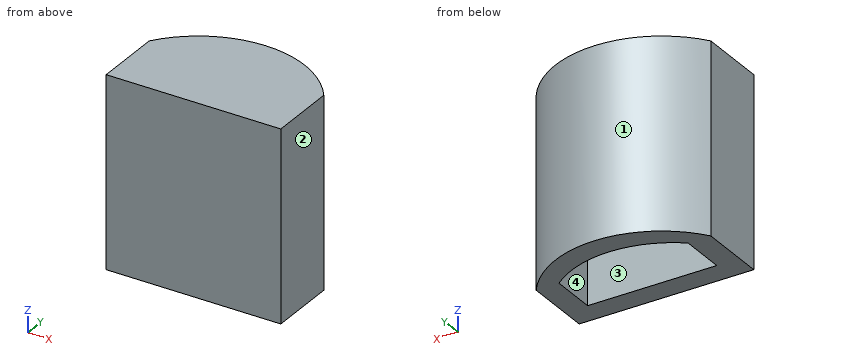
from build123d import *

# Parameters (mm, degrees)
EXTRUDE_1_DEPTH      = 5
EXTRUDE_2_DEPTH      = 5
EXTRUDE_2_DEPTH_BACK = 20


with BuildPart() as part:
    # 草圖1 → 填料-伸長1 (new body)
    with BuildSketch(Plane.XY):
        with BuildLine():
            Line((-8.181868209, 3.138333333), (-8.181868209, -2.861666667))
            Line((-8.181868209, -2.861666667), (8.818131791, -2.861666667))
            Line((8.818131791, -2.861666667), (8.818131791, 3.138333333))
            ThreePointArc((8.818131791, 3.138333333), (0.318131791, 6.138333333), (-8.181868209, 3.138333333))
        make_face()
    extrude(amount=EXTRUDE_1_DEPTH)

    # 草圖1<4> → 填料-伸長2 (add, two sides: drawn at the far end of the back side and taken through both)
    with BuildSketch(Plane.XY.offset(-EXTRUDE_2_DEPTH_BACK)):
        with BuildLine():
            Line((-11.181868209, 3.138333333), (-11.181868209, -5.861666667))
            Line((-11.181868209, -5.861666667), (11.818131791, -5.861666667))
            Line((11.818131791, -5.861666667), (11.818131791, 3.138333333))
            ThreePointArc((11.818131791, 3.138333333), (0.318131791, 9.138333333), (-11.181868209, 3.138333333))
        make_face()
        with BuildLine():
            Line((-8.181868209, 3.138333333), (-8.181868209, -2.861666667))
            Line((-8.181868209, -2.861666667), (8.818131791, -2.861666667))
            Line((8.818131791, -2.861666667), (8.818131791, 3.138333333))
            ThreePointArc((8.818131791, 3.138333333), (0.318131791, 6.138333333), (-8.181868209, 3.138333333))
        make_face(mode=Mode.SUBTRACT)
    extrude(amount=EXTRUDE_2_DEPTH + EXTRUDE_2_DEPTH_BACK)


solid = part.part
Part model, mm, in its own coordinate system. Face numbers are marked on the shaded views. Round coordinates to 2 decimals unless told otherwise and drop trailing zeros. Loops run counter-clockwise (first coordinate to the right, second up) from the corner with the lowest first, then second, coordinate; pieces in that order, holes last. Notation, with made-up numbers: (83, 50.5) - (95, 50.5) arc R21 cw to (95, 69.5) - close; hole circle Ø8 at (64.25, 20). An arc over 180 degrees is marked (long way). Answer as a JSON object with one key per item and string values.
Item 1: Pull direction Y, two halves, no side cores. Call the marked faces 1, 2, 3 and 4: pulls with the +Y half, pulls with the -Y half, needs draft (parallel to the pull), parting line crosses it, or undercut.
Output:
{"face 1": "pulls with the +Y half", "face 2": "needs draft", "face 3": "undercut", "face 4": "undercut"}
Item 2: Band-saw the part on D-D on z = 0.5. List the corners of the cut face in (x, y).
Output:
{"outline": "(-11.18, -5.86) - (11.82, -5.86) - (11.82, 3.14) arc R14.02 ccw to (-11.18, 3.14) - close"}
Item 3: Wall check: L1, parallel to X at y = 1.25, z = -1.75; L2, parallel to Y at x = -7.25, z = -2.25; L3, parallel to Z at x = -5.5, y = 4. Give the ranges that are in metal, low to high.
Output:
{"L1": "-11.18 to -8.18, 8.82 to 11.82", "L2": "-5.86 to -2.86, 3.83 to 6.92", "L3": "0 to 5"}
Item 4: Band-saw the part on B-B on x = 6.25. List the corners of the cut face in (y, z), plus the area to 3 significant figures.
Output:
{"outline": "(-5.86, -20) - (-2.86, -20) - (-2.86, 0) - (4.77, 0) - (4.77, -20) - (7.82, -20) - (7.82, 5) - (-5.86, 5) - close", "area": "189 mm2"}
Item 5: Band-saw the part on C-C on y = -1.5. List the corners of the cut face in (x, z).
Output:
{"outline": "(-11.18, -20) - (-8.18, -20) - (-8.18, 0) - (8.82, 0) - (8.82, -20) - (11.82, -20) - (11.82, 5) - (-11.18, 5) - close"}
Item 6: Pin check, flat tips, straight feed: pin 1 (1 mm diameter, centred on y = 6, z = 1.5, fed in from +X); pin 2 (4 mm diameter, centred on x = -7, z = -11, fed in from +Y); pin 3 (7 mm diameter, centred on x = 1.5, y = -0.5, fed in from -Z). Stop position of each tip, or through.
Output:
{"pin 1": "x = 9.74", "pin 2": "y = 8.09", "pin 3": "z = -20"}
Item 7: Band-saw the part on A-A on z = -16. List the corners of the cut face in (x, y).
Output:
{"outline": "(-11.18, -5.86) - (11.82, -5.86) - (11.82, 3.14) arc R14.02 ccw to (-11.18, 3.14) - close; hole (-8.18, -2.86) - (8.82, -2.86) - (8.82, 3.14) arc R13.54 ccw to (-8.18, 3.14) - close"}
